Work out the finished part from the listing and answer in its coordinate system (mm). Face numbers are marked on the shaded views. A direction names the side the tool comes from. Give positions to 0.01 mm unless a question says otherwise; leave off trailing zeros. Write each loop counter-clockwise with the first axis right and the second up, starting at its lowest first coordinate (ties: lowest second). Pieces come first, ordered by that corner, then holes. Notation, with made-up numbers: (-15, 48) - (41, 48) arc R23 ccw to (41, 74) - close; hole circle Ø11 at (-28.75, -16). An arc over 180 degrees is marked (long way). Write each question's results on one line, items separated by ' | '. Start each with the question number.
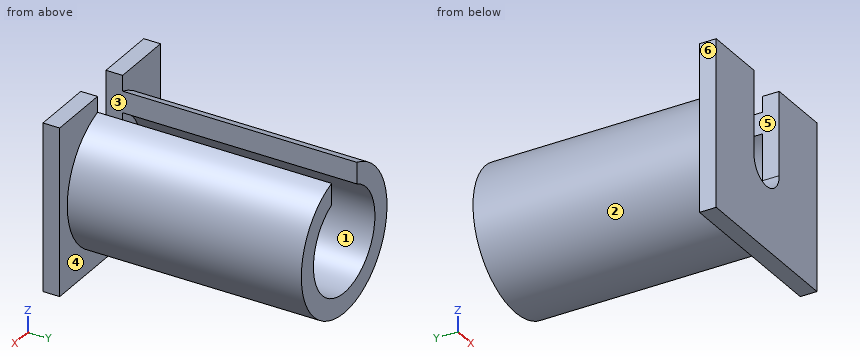
from build123d import *

# Parameters (mm, degrees)
SKETCH1_R           = 4.25
SKETCH1_R_2         = 3.05
BOSS_EXTRUDE1_DEPTH = 15
SKETCH2_R           = 3.05
SKETCH2_R_2         = 1.25
BOSS_EXTRUDE2_DEPTH = 1
CUT_EXTRUDE1_DEPTH  = 15
BOSS_EXTRUDE3_DEPTH = 1


with BuildPart() as part:
    # Sketch1 → Boss-Extrude1 (new body)
    with BuildSketch(Plane(origin=(0, 0, 0), x_dir=(1, 0, 0), z_dir=(0, 1, 0))):
        with Locations(Location((0, 0, 0), (0, 0, 270))):
            Circle(SKETCH1_R)
        with Locations(Location((0, 0, 0), (0, 0, 270))):
            Circle(SKETCH1_R_2, mode=Mode.SUBTRACT)
    extrude(amount=BOSS_EXTRUDE1_DEPTH)

    # Sketch2 → Boss-Extrude2 (add)
    with BuildSketch(Plane(origin=(0, 0, 0), x_dir=(1, 0, 0), z_dir=(0, 1, 0))):
        with Locations(Location((0, 0, 0), (0, 0, 270))):
            Circle(SKETCH2_R)
        with Locations(Location((0, 0, 0), (0, 0, 270))):
            Circle(SKETCH2_R_2, mode=Mode.SUBTRACT)
    extrude(amount=BOSS_EXTRUDE2_DEPTH)

    # Sketch3 → Cut-Extrude1 (cut)
    with BuildSketch(Plane(origin=(0, 0, 0), x_dir=(1, 0, 0), z_dir=(0, 1, 0))):
        with BuildLine():
            ThreePointArc((1.25, 0), (0, -1.25), (-1.25, 0))
            Line((-1.25, 0), (-1.25, -5.072282681))
            Line((-1.25, -5.072282681), (1.25, -5.072282681))
            Line((1.25, -5.072282681), (1.25, 0))
        make_face()
    extrude(amount=CUT_EXTRUDE1_DEPTH, mode=Mode.SUBTRACT)

    # Sketch4 → Boss-Extrude3 (add)
    with BuildSketch(Plane(origin=(0, 0, 0), x_dir=(1, 0, 0), z_dir=(0, 1, 0))):
        with BuildLine():
            Line((-1.25, -5), (-1.25, 0))
            ThreePointArc((-1.25, 0), (0, 1.25), (1.25, 0))
            Line((1.25, 0), (1.25, -5))
            Line((1.25, -5), (5, -5))
            Line((5, -5), (5, 5))
            Line((5, 5), (-5, 5))
            Line((-5, 5), (-5, -5))
            Line((-5, -5), (-1.25, -5))
        make_face()
    extrude(amount=BOSS_EXTRUDE3_DEPTH)


solid = part.part
Q1. A tool of negligible diameter and unlimited length cuts with its end or side. For the marked faces 5 and 6, from which of +Z, -Z, +X, -X, +Y, -Y can it reach the whole face along a straight path? Write none if from no direction.
Q2. A cutting plane is placed at D-D, the plane y = 8.5. Write down the section's boundary in (x, z), and give its area (3 significant figures).
Q3. A cutting plane is placed at C-C, the plane z = -3.5. Write down the section's boundary in (x, y), and give its area (3 significant figures).
Q4. Consider L1, parallel to X at y = 4.5, z = 0; L2, parallel to Z at x = 0, y = 10.5; L3, parallel to Y at x = 2, z = 0.5. Determine where each line is inside the solid, lowest interval first.
Q5. The mould has two halves that part along X. Classify the marked faces 1, 2, 3 and 4: pulls with the +X half, pulls with the -X half, needs draft (parallel to the pull), parting line crosses it, or undercut.
Q6. A cutting plane is placed at A-A, the plane z = 1.5. Write down the section's boundary in (x, y).
Q7. Given pin 1 (1.5 mm diameter, centred on x = 2, z = 1.5, fed in from -Y); pin 2 (2 mm diameter, centred on x = -1.5, y = 11, fed in from +Z); pin 3 (5.5 mm diameter, centred on y = 5, z = 1.5, fed in from -X); pin 4 (1.7 mm diameter, centred on x = 0.5, z = -0.5, fed in from +Y), each flat-ended and moving along its own axis, determine where each tip first touches the part or whether it passes through.
Q8. A cutting plane is placed at B-B, the plane x = 3.75. Write down the section's boundary in (y, z), and give its area (3 significant figures).
Result:
1) face 5: +Z, +Y, -Y | face 6: +Z, -Z, -X, +Y, -Y
2) outline: (-1.25, 2.78) - (-1.25, 4.06) arc R4.25 ccw (long way) to (1.25, 4.06) - (1.25, 2.78) arc R3.05 cw (long way) to start | area: 24.5 mm2
3) outline: (-5, 0) - (5, 0) - (5, 1) - (2.41, 1) - (2.41, 15) - (-2.41, 15) - (-2.41, 1) - (-5, 1) - close | area: 77.5 mm2
4) L1: x = -4.25 to -3.05, 3.05 to 4.25 | L2: z = -4.25 to -3.05 | L3: y = 0 to 1
5) face 1: undercut | face 2: parting line crosses it | face 3: undercut | face 4: needs draft
6) outline: (-5, 0) - (-1.25, 0) - (-1.25, 1) - (-2.66, 1) - (-2.66, 15) - (-3.98, 15) - (-3.98, 1) - (-5, 1) - close; (1.25, 0) - (5, 0) - (5, 1) - (3.98, 1) - (3.98, 15) - (2.66, 15) - (2.66, 1) - (1.25, 1) - close
7) pin 1: stops at y = 0 | pin 2: stops at z = 4.06 | pin 3: stops at x = -4.25 | pin 4: stops at y = 1
8) outline: (0, -5) - (1, -5) - (1, -2) - (15, -2) - (15, 2) - (1, 2) - (1, 5) - (0, 5) - close | area: 66.0 mm2
